Build history of the part. All positions in model axes, mm. Give positions to 0.01 mm unless a question says otherwise; leave off trailing zeros. Order: outer loops, then holes, each group sorted by start corner. A loop starts at its lowest first (then second) coordinate and runs counter-clockwise, first axis right, second up. Notation, with made-up numbers: (-16.5, 58.25) -> (-0.5, 58.25) arc R27 cw to (-0.5, 82.25) -> close; hole circle Ø6 at (67.5, 60). An arc over 180 degrees is marked (long way). One line per question, with ' | ' between items. Start each with the question number.
(1) Drill centre lines: L1, parallel to Y at x = 0, z = 38; L2, parallel to Z at x = -16, y = -0.5; L3, parallel to Y at x = 1.5, z = 42. Where is each one in solid material? Low to high. Write a range as from..to.
(2) Cut at C-C (z = 118). Give the cut face in (x, y), then the cut area to 3 significant figures.
(3) Pin check, flat tips, straight feed: pin 1 Ø10 at (x, z) = (15.5, 39) entering from -Y; pin 2 Ø1 at (x, z) = (-27, 67.5) entering from +Y; pin 3 Ø5 at (y, z) = (-25, 106.5) entering from -X. Stop position of each tip, or through.
(4) Cut at A-A (x = 0). Give the cut face in (y, z) (3 decimals), then the cut area to 3 significant figures.
(5) Pull direction X, two halves, no side cores. Call faces 1 (the face through (-1, 1, 0)), 2 (the face through (-30.235, -23.183, 61.077)), 3 (the face through (-7.709, -34.714, 63.899)): +X half, -X half, draft (parallel to the pull), parting line (faces both ways), or undercut.
from build123d import *

# Parameters (mm, degrees)
F0_R     = 38.1
F1_DEPTH = 127
F2_T     = -2.54


# Not quite as in the source:
# - a fillet or chamfer that OpenCascade refuses, or shapes differently, is made with other operations: its cross-section is extruded or revolved along the edge and cut away or added


with BuildPart() as f1:
    # F0 (on Top) → F1 (new body)
    with BuildSketch(Plane.XY):
        Circle(F0_R)
    extrude(amount=F1_DEPTH)

    # F2
    f2_openings = [f1.faces().sort_by_distance(p)[0] for p in [
        (0, 0, 127),
    ]]
    offset(amount=F2_T, openings=f2_openings)

    # F3: fillet of radius 3.175 on 1 edges, made by hand

    # F3_s1 → F3_t2 (revolve, cut)
    with BuildSketch(Plane.XZ):
        with BuildLine():
            ThreePointArc((38.1, 123.8891480267), (37.3843444248, 125.8971943409), (35.56, 127))
            Line((35.56, 127), (38.1, 127))
            Line((38.1, 127), (38.1, 123.8891480267))
        make_face()
    revolve(axis=Axis((0, 0, 127), (0, 0, 1)), mode=Mode.SUBTRACT)


solid = f1.part
Result set:
1) L1: y = -38.1..-35.56, 35.56..38.1 | L2: z = 0..2.54 | L3: y = -38.07..-35.53, 35.53..38.07
2) outline: circle Ø76.2 at (0, 0); hole circle Ø71.12 at (0, 0) | area: 588 mm2
3) pin 1: stops at y = -36.62 | pin 2: stops at y = 27.37 | pin 3: stops at x = -30.75
4) outline: (-38.1, 0) -> (38.1, 0) -> (38.1, 123.889) arc R3.175 ccw to (35.56, 127) -> (35.56, 2.54) -> (-35.56, 2.54) -> (-35.56, 127) arc R3.175 ccw to (-38.1, 123.889) -> close | area: 822 mm2
5) face 1: draft | face 2: parting line | face 3: undercut
